The listing builds one solid part. Answer for the finished solid, in the listing's coordinates (mm). A direction names the side the tool comes from. Give positions to 0.01 mm unless a question says otherwise; leave off trailing zeros. Order: outer loops, then holes, each group sorted by start corner. A loop starts at its lowest first (then second) coordinate and runs counter-clockwise, first axis right, second up. Notation, with made-up numbers: (10.25, 65) - (63.25, 65) arc R28 cw to (63.25, 93) - close; hole circle Ø9 at (-23, 54.25). An arc over 180 degrees is marked (long way). Write each question's results on one line, items separated by ' | '. Start each with the question number.
1. Determine the mould class of faces 1 (the face through (2.51, -8.056, -2.86)), 2 (the face through (0, -5, 11.7)), 3 (the face through (2.6, 3.4, 2.05)), 4 (the face through (2.6, 3.4, -2.05)) for opening direction Z: released by +Z, released by -Z, zero draft, split by the parting line, or undercut.
2. Flat-ended cylindrical pins translate along their axes: pin 1 (4 mm diameter, centred on x = 2.5, z = 8, fed in from +Y); pin 2 (1 mm diameter, centred on x = 2, z = -1, fed in from +Y); pin 3 (1.2 mm diameter, centred on x = 2.5, y = 3.5, fed in from -Z). Find the tip coordinate at first contact, or state that the pin passes through.
3. Section B-B (y = 2) is taken. Give the vertices of the cut face in (x, z) (3 decimals), and give its area (3 significant figures).
4. Section A-A (y = -4.9) is taken. Give the vertices of the cut face in (x, z).
5. Find the intervals of material crossed by L1, parallel to Z at x = 2.75, y = -5.25; L2, parallel to Z at x = 0, y = 0.75; L3, parallel to Y at x = -3, z = 0, in increasing order.
6. Section C-C (x = 1.25) is taken. Give the vertices of the cut face in (y, z), and give its area (3 significant figures).
7. Section D-D (z = 2.25) is taken. Give the vertices of the cut face in (x, y).
8. Which of the six approach directions +Z, -Z, +X, -X, +Y, -Y give full straight-line access (tool end or side, diameter ignored) to faces 5 (the face through (2.5, 3.6, -3.05)), 6 (the face through (-3, 0, 3)), 7 (the face through (0.5, -7.7, 6.1)), 8 (the face through (3, 0, 3))?
from build123d import *

# Parameters (mm, degrees)
SKETCH1_W           = 7
SKETCH1_H           = 7
BOSS_EXTRUDE1_DEPTH = 1.3
SKETCH2_W           = 1.45
SKETCH2_H           = 1.45
BOSS_EXTRUDE2_DEPTH = 0.4
SKETCH3_W           = 1
SKETCH3_H           = 1
BOSS_EXTRUDE3_DEPTH = 3.9
SKETCH4_R           = 0.625
BOSS_EXTRUDE4_DEPTH = 4.2
SKETCH5_R           = 3.5
BOSS_EXTRUDE5_DEPTH = 1.2
SKETCH6_W           = 7
SKETCH6_H           = 7
BOSS_EXTRUDE6_DEPTH = 7.1
CHAMFER1_START      = 8.88850564
CHAMFER1_OUTLINE_W  = 6
CHAMFER1_OUTLINE_H  = 6
CHAMFER1_DEPTH      = 2.11149436
CHAMFER2_START      = -11
CHAMFER2_OUTLINE_W  = 6
CHAMFER2_OUTLINE_H  = 6
CHAMFER2_DEPTH      = 2.11149436
CHAMFER3_START      = 8.88850564
CHAMFER3_OUTLINE_W  = 6
CHAMFER3_OUTLINE_H  = 6
CHAMFER3_DEPTH      = 2.11149436
CHAMFER4_START      = -11
CHAMFER4_OUTLINE_W  = 6
CHAMFER4_OUTLINE_H  = 6
CHAMFER4_DEPTH      = 2.11149436
CHAMFER5_SIZE       = 0.3
SKETCH7_R           = 3.1
BOSS_EXTRUDE7_DEPTH = 2.6
SKETCH8_R           = 2.68986
BOSS_EXTRUDE8_DEPTH = 5.6


with BuildPart() as part:
    # Sketch1 → Boss-Extrude1 (new body)
    with BuildSketch(Plane(origin=(0, 0, 0), x_dir=(1, 0, 0), z_dir=(0, 1, 0))):
        Rectangle(SKETCH1_W, SKETCH1_H)
    extrude(amount=BOSS_EXTRUDE1_DEPTH)

    # Sketch2 → Boss-Extrude2 (add)
    with BuildSketch(Plane(origin=(0, 1.3, 0), x_dir=(1, 0, 0), z_dir=(0, 1, 0))):
        with Locations((-2.775, 2.775)):
            Rectangle(SKETCH2_W, SKETCH2_H)
        with Locations((2.775, 2.775)):
            Rectangle(SKETCH2_W, SKETCH2_H)
        with Locations((2.775, -2.775)):
            Rectangle(SKETCH2_W, SKETCH2_H)
        with Locations((-2.775, -2.775)):
            Rectangle(SKETCH2_W, SKETCH2_H)
    extrude(amount=BOSS_EXTRUDE2_DEPTH)

    # Sketch3 → Boss-Extrude3 (add)
    with BuildSketch(Plane(origin=(0, 1.7, 0), x_dir=(1, 0, 0), z_dir=(0, 1, 0))):
        with Locations((-2.55, 2.55)):
            Rectangle(SKETCH3_W, SKETCH3_H)
        with Locations((-2.55, -2.55)):
            Rectangle(SKETCH3_W, SKETCH3_H)
        with Locations((2.55, -2.55)):
            Rectangle(SKETCH3_W, SKETCH3_H)
        with Locations((2.55, 2.55)):
            Rectangle(SKETCH3_W, SKETCH3_H)
    extrude(amount=BOSS_EXTRUDE3_DEPTH)

    # Sketch4 → Boss-Extrude4 (add)
    with BuildSketch(Plane(origin=(0, 1.3, 0), x_dir=(1, 0, 0), z_dir=(0, 1, 0))):
        with Locations(Location((0, 0, 0), (0, 0, 270))):
            Circle(SKETCH4_R)
    extrude(amount=BOSS_EXTRUDE4_DEPTH)

    # Sketch5 → Boss-Extrude5 (add)
    with BuildSketch(Plane(origin=(0, 0, 0), x_dir=(-1, 0, 0), z_dir=(0, -1, 0))):
        with Locations(Location((0, 0, 0), (0, 0, 90))):
            Circle(SKETCH5_R)
    extrude(amount=BOSS_EXTRUDE5_DEPTH)

    # Sketch6 → Boss-Extrude6 (add)
    with BuildSketch(Plane(origin=(0, -1.2, 0), x_dir=(-1, 0, 0), z_dir=(0, -1, 0))):
        Rectangle(SKETCH6_W, SKETCH6_H)
    extrude(amount=BOSS_EXTRUDE6_DEPTH)

    # Chamfer1: read off the stored shape, not the designer's step
    # Chamfer1 outline → Chamfer1 (cut)
    with BuildSketch(Plane(origin=(0, 0, 0), x_dir=(0.9655189447347837, 0.25069112066556, 0.07019351378635694), z_dir=(0.26033280115696106, -0.9297600041320021, -0.26033280115696106)).offset(CHAMFER1_START)):
        Rectangle(CHAMFER1_OUTLINE_W, CHAMFER1_OUTLINE_H)
    extrude(amount=CHAMFER1_DEPTH, mode=Mode.SUBTRACT)

    # Chamfer2: read off the stored shape, not the designer's step
    # Chamfer2 outline → Chamfer2 (cut)
    with BuildSketch(Plane(origin=(0, 0, 0), x_dir=(0.9655189447347837, -0.25069112066556, -0.07019351378635694), z_dir=(0.26033280115696106, 0.9297600041320021, 0.26033280115696106)).offset(CHAMFER2_START)):
        Rectangle(CHAMFER2_OUTLINE_W, CHAMFER2_OUTLINE_H)
    extrude(amount=CHAMFER2_DEPTH, mode=Mode.SUBTRACT)

    # Chamfer3: read off the stored shape, not the designer's step
    # Chamfer3 outline → Chamfer3 (cut)
    with BuildSketch(Plane(origin=(0, 0, 0), x_dir=(0.9655189447347837, 0.25069112066556, -0.07019351378635694), z_dir=(0.26033280115696106, -0.9297600041320021, 0.26033280115696106)).offset(CHAMFER3_START)):
        Rectangle(CHAMFER3_OUTLINE_W, CHAMFER3_OUTLINE_H)
    extrude(amount=CHAMFER3_DEPTH, mode=Mode.SUBTRACT)

    # Chamfer4: read off the stored shape, not the designer's step
    # Chamfer4 outline → Chamfer4 (cut)
    with BuildSketch(Plane(origin=(0, 0, 0), x_dir=(0.9655189447347837, -0.25069112066556, 0.07019351378635694), z_dir=(0.26033280115696106, 0.9297600041320021, -0.26033280115696106)).offset(CHAMFER4_START)):
        Rectangle(CHAMFER4_OUTLINE_W, CHAMFER4_OUTLINE_H)
    extrude(amount=CHAMFER4_DEPTH, mode=Mode.SUBTRACT)

    # Chamfer5
    chamfer5_edges = [part.edges().sort_by_distance(p)[0] for p in [
        (3.5, 0.85, 3.5),
        (-3.5, 0.85, 3.5),
        (-3.5, 0.85, -3.5),
        (3.5, 0.85, -3.5),
    ]]
    chamfer(chamfer5_edges, length=CHAMFER5_SIZE)

    # Sketch7 → Boss-Extrude7 (add)
    with BuildSketch(Plane.XY.offset(3.5)):
        with Locations(Location((0, -4.9, 0), (0, 0, 180))):
            Circle(SKETCH7_R)
    extrude(amount=BOSS_EXTRUDE7_DEPTH)

    # Sketch8 → Boss-Extrude8 (add)
    with BuildSketch(Plane.XY.offset(6.1)):
        with Locations((0, -4.9)):
            Circle(SKETCH8_R)
    extrude(amount=BOSS_EXTRUDE8_DEPTH)


solid = part.part
Reported:
1) face 1: released by -Z | face 2: released by +Z | face 3: undercut | face 4: undercut
2) pin 1: y = -2.26 | pin 2: y = 1.3 | pin 3: z = -3.05
3) outline: (-3.05, -3.05) - (-2.05, -3.05) - (-2.05, -2.05) - (-3.05, -2.05) - close; (-3.05, 2.05) - (-2.05, 2.05) - (-2.05, 3.05) - (-3.05, 3.05) - close; circle Ø1.25 at (0, 0); (2.05, -3.05) - (3.05, -3.05) - (3.05, -2.05) - (2.05, -2.05) - close; (2.05, 2.05) - (3.05, 2.05) - (3.05, 3.05) - (2.05, 3.05) - close | area: 5.23 mm²
4) outline: (-3.5, -3.5) - (3.5, -3.5) - (3.5, 3.5) - (3.1, 3.5) - (3.1, 6.1) - (2.69, 6.1) - (2.69, 11.7) - (-2.69, 11.7) - (-2.69, 6.1) - (-3.1, 6.1) - (-3.1, 3.5) - (-3.5, 3.5) - close
5) L1: -3.5 to 6.1 | L2: -3.5 to 3.5 | L3: -8.3 to 1.3
6) outline: (-8.3, -3.25) - (-8.23, -3.5) - (-1.2, -3.5) - (-1.2, -3.27) - (0, -3.27) - (0, -3.5) - (1.3, -3.5) - (1.3, 3.5) - (0, 3.5) - (0, 3.27) - (-1.2, 3.27) - (-1.2, 3.5) - (-2.06, 3.5) - (-2.06, 6.1) - (-2.52, 6.1) - (-2.52, 11.7) - (-7.28, 11.7) - (-7.28, 6.1) - (-7.74, 6.1) - (-7.74, 3.5) - (-8.23, 3.5) - (-8.3, 3.25) - close | area: 108 mm²
7) outline: (-3.5, -7.95) - (-2.25, -8.3) - (2.25, -8.3) - (3.5, -7.95) - (3.5, -1.2) - (2.68, -1.2) - (2.68, 0) - (3.5, 0) - (3.5, 1.7) - (3.05, 1.7) - (3.05, 5.6) - (2.05, 5.6) - (2.05, 1.3) - (-2.05, 1.3) - (-2.05, 5.6) - (-3.05, 5.6) - (-3.05, 1.7) - (-3.5, 1.7) - (-3.5, 0) - (-2.68, 0) - (-2.68, -1.2) - (-3.5, -1.2) - close
8) face 5: -Z, +X, -X, +Y | face 6: +Z, -X | face 7: +Z | face 8: +Z, +X
